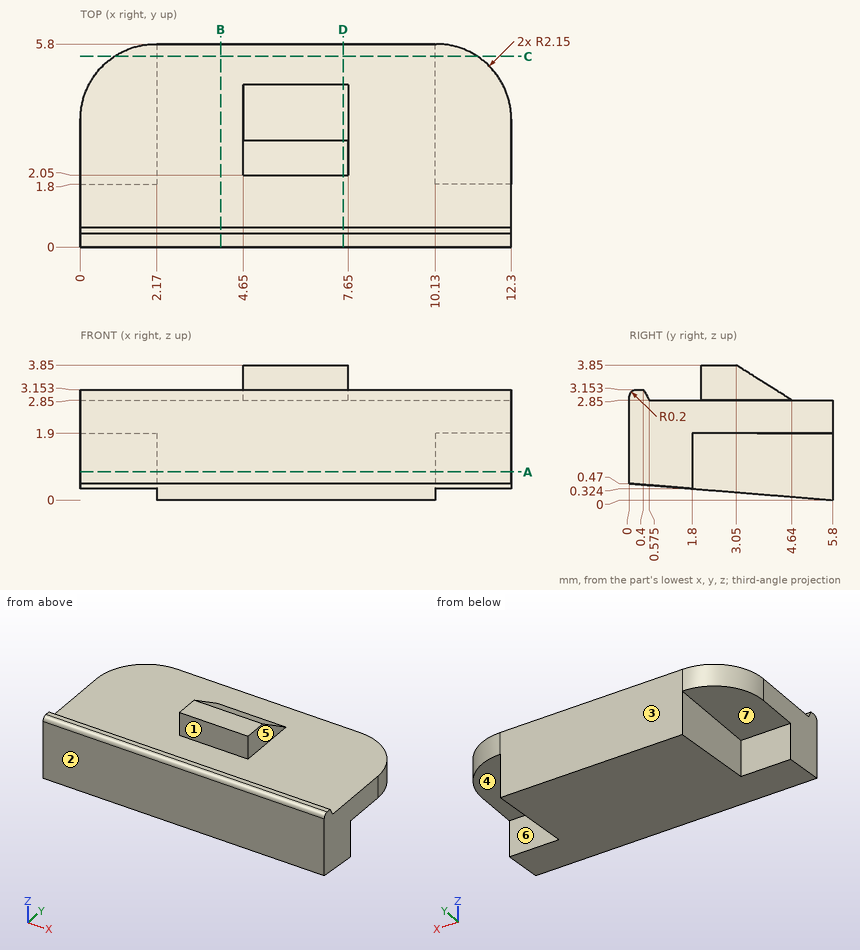
The figure shows three views and two pictorial views of one solid part (mm, origin at its lowest corner). Answer the questions. A direction names the side the tool comes from. Give positions to 0.01 mm unless a question says otherwise; leave off trailing zeros. Write each loop counter-clockwise with the first axis right and the second up, starting at its lowest first coordinate (ties: lowest second). Pieces come first, ordered by that corner, then holes. Notation, with made-up numbers: (-12, 24.5) - (6, 24.5) arc R26 cw to (6, 44.5) - close; hole circle Ø3 at (5, 56.5). An arc over 180 degrees is marked (long way). Return JSON: item names as keys, results as strings.
Q1. A cutting plane is placed at A-A, the plane z = 0.8. Determine the outline of the cut face in (x, y), and give its area (3 significant figures).
Reply:
{"outline": "(0, 0) - (12.3, 0) - (12.3, 1.8) - (10.13, 1.8) - (10.13, 5.8) - (2.17, 5.8) - (2.17, 1.8) - (0, 1.8) - close", "area": "54.0 mm²"}
Q2. A cutting plane is placed at B-B, the plane x = 4. Determine the outline of the cut face in (y, z) (3 decimals).
Reply:
{"outline": "(0, 0.47) - (5.8, 0) - (5.8, 2.85) - (0.575, 2.85) - (0.4, 3.153) - (0.2, 3.153) arc R0.2 ccw to (0, 2.953) - close"}
Q3. For the marked faces 5, 6 and 7, determine the directions among +Z, -Z, +X, -X, +Y, -Y from which every point of the face is accessible in a straight line to the end or side of a thin tool.
Reply:
{"face 5": "+Z, +X, +Y", "face 6": "-Z, +X, +Y", "face 7": "-Z, -X, +Y"}
Q4. Given P1, Ø1.6, axis at x = 9, y = 3, coming from the +Z side; P2, Ø1, axis at x = 10.5, y = 3.5, coming from the -Z side; P3, Ø0.5, axis at x = 11, z = 1, coming from the +Y side, each flat-ended and moving along its own axis, determine where each tip first touches the part or whether it passes through.
Reply:
{"P1": "z = 2.85", "P2": "z = 0.16", "P3": "y = 1.8"}
Q5. A cutting plane is placed at C-C, the plane y = 5.45. Determine the outline of the cut face in (x, z).
Reply:
{"outline": "(0.97, 1.9) - (2.17, 1.9) - (2.17, 0.03) - (10.13, 0.03) - (10.13, 1.9) - (11.33, 1.9) - (11.33, 2.85) - (0.97, 2.85) - close"}
Q6. For a pull along Y with two mould halves and no side action, classify the marked faces 1, 2, 3 and 4 as released by +Y, released by -Y, zero draft, split by the parting line, or undercut.
Reply:
{"face 1": "undercut", "face 2": "released by -Y", "face 3": "released by +Y", "face 4": "zero draft"}
Q7. Consider line 1 along Z through (x, y) = (1, 2.95); line 2 along X through (y, z) = (4.25, 1.5); line 3 along Y through (x, z) = (11.25, 0.8). Determine where each line is inside the solid, lowest interval first. Write a range as [from, to].
Reply:
{"line 1": "[1.9, 2.85]", "line 2": "[2.17, 10.13]", "line 3": "[0, 1.8]"}
Q8. A cutting plane is placed at D-D, the plane x = 7.5. Determine the outline of the cut face in (y, z) (3 decimals).
Reply:
{"outline": "(0, 0.47) - (5.8, 0) - (5.8, 2.85) - (4.64, 2.85) - (3.05, 3.85) - (2.05, 3.85) - (2.05, 2.85) - (0.575, 2.85) - (0.4, 3.153) - (0.2, 3.153) arc R0.2 ccw to (0, 2.953) - close"}
